Part model, mm, in its own coordinate system. A direction names the side the tool comes from. Round coordinates to 2 decimals unless told otherwise and drop trailing zeros. Loops run counter-clockwise (first coordinate to the right, second up) from the corner with the lowest first, then second, coordinate; pieces in that order, holes last. Notation, with made-up numbers: (9.5, 69) -> (33.5, 69) arc R18 ccw to (33.5, 84) -> close; hole circle Ø7 at (25, -12.75). An arc over 180 degrees is marked (long way). Answer as a JSON object with one key per item and string values. Group by question number.
Autodesk Inventor part; units mm, degrees
ref_plane "YZ Plane" through (0, 0, 0) normal (1, 0, 0) x (0, 1, 0)
ref_plane "XZ Plane" through (0, 0, 0) normal (0, 1, 0) x (-1, 0, 0)
ref_plane "XY Plane" through (0, 0, 0) normal (0, 0, 1) x (1, 0, 0)
sketch "Sketch1" plane through (0, 0, 0) normal (0, 1, 0) x (-1, 0, 0)
  line L0 (0, 0) -> (0, 25.4)
  line L1 (0, 25.4) -> (50.8, 25.4)
  line L2 (50.8, 25.4) -> (50.8, 0)
  line L3 (50.8, 0) -> (0, 0)
  dimension "d0" = 25.4
  dimension "d1" = 50.8
extrude "Plate1" add sketch "Sketch1" along normal blind 3.048
sketch "Sketch2" plane through (-3.048, 0, 0) normal (1, 0, 0) x (0, 1, 0)
  line L0 (0, 25.4) -> (0, 0)
  line L1 (0, 0) -> (76.2, 0)
  line L2 (76.2, 0) -> (76.2, 25.4)
  line L3 (76.2, 25.4) -> (0, 25.4)
edge flange "Flange1" height 76.2 angle 90 thickness 3.048 bend radius 3.048 thickness toward (1, 0, 0) relief tear relief width 3.048 relief depth 1.524 edges at (0, 3.048, 12.7) wall of the first edge with corners at (-3.048, 0, 25.4) (-3.048, 0, 0) (-3.048, 76.2, 0) (-3.048, 76.2, 25.4)
bend "Bend1"
corner "Corner1"
hole "Hole1" at (-3.048, 12.7, 12.7) direction (1, 0, 0) diameter 6.35 end through all
pattern_linear "Rectangular Pattern1" count 3 spacing 25.4 along (0, 1, 0) of "Hole1"
hole "Hole2" at (-12.7, 3.048, 12.7) direction (0, -1, 0) diameter 6.35 end through all
pattern_linear "Rectangular Pattern2" count 2 spacing 25.4 along (-1, 0, 0) of "Hole2"
equation "\"d20\" = Thickness"
equation "\"d32\" = Thickness"
equation "\"d3\" = BendReliefWidth"
equation "\"d4\" = BendReliefDepth"
equation "\"d5\" = MinimumRemnant"
equation "\"d6\" = BendRadius"
equation "\"d9\" = BendRadius"
equation "\"d10\" = CornerReliefSize"
equation "\"d11\" = GapSize"
equation "\"d12\" = JacobiRadiusSize"
equation "\"BendRadius\" = Thickness"
equation "\"BendReliefWidth\" = Thickness"
equation "\"BendReliefDepth\" = 0.5 * Thickness"
equation "\"CornerReliefSize\" = 4 * Thickness"
equation "\"MinimumRemnant\" = 2 * Thickness"
equation "\"TransitionRadius\" = BendRadius"
equation "\"JacobiRadiusSize\" = BendRadius"
equation "\"GapSize\" = Thickness"
equation "\"d2\" = BendRadius"
properties part number "L-Gusset Steel Plate"
Item 1: Band-saw the part on A-A, the plane x = -38.1. List the corners of the cut face in (y, z) (3 decimals), plus the area to 3 significant figures.
Item 2: Band-saw the part on C-C, the plane z = 12.7. List the corners of the cut face in (x, y) (3 decimals), plus the area to 3 significant figures.
Item 3: Band-saw the part on B-B, the plane y = 12.7. List the corners of the cut face in (x, z) (3 decimals), plus the area to 3 significant figures.
Item 4: Two-plate mould, pull along Y, no slides. Class faces 3 (the face through (-1.5, 14.63, 10.18)), 4 (the face through (-2, 76.2, 13)), 5 (the face through (-50.8, 2, 13)), 6 (the face through (-1.503, 61.354, 10.36)): pulls with the +Y half, pulls with the -Y half, needs draft (parallel to the pull), parting line crosses it, or undercut.
Item 5: Band-saw the part on D-D, the plane z = 5.5. List the corners of the cut face in (x, y), plus the area to 3 significant figures.
Item 6: Drill centre lines: line 1 (Y direction, x = -1.75, z = 12.7) (3 decimals); line 2 (Z direction, x = -0.7, y = 38.1) (3 decimals); line 3 (X direction, y = 2, z = 12.7) (3 decimals). Where is each one in solid material? Low to high.
Item 7: Which spindle directions (+Z, -Z, +X, -X, +Y, -Y) get a long thin tool onto all of the face, cutting with end or side? Do faces 1 (the face through (-2.7, 27, 0)), 2 (the face through (-3.048, 41, 15)). Say none if no direction does.
Item 8: Drop flat-ended pins along their axis: pin 1 Ø12.5 at (y, z) = (40.5, 14) entering from -X; pin 2 Ø8 at (x, z) = (-27.5, 16.5) entering from +Y. Give the stop position or say it passes through.
Entries:
{
 "1": {"outline": "(0, 0) -> (3.048, 0) -> (3.048, 9.525) -> (0, 9.525) -> close; (0, 15.875) -> (3.048, 15.875) -> (3.048, 25.4) -> (0, 25.4) -> close", "area": "58.1 mm²"},
 "2": {"outline": "(-50.8, 0) -> (-41.275, 0) -> (-41.275, 3.048) -> (-50.8, 3.048) -> close; (-34.925, 0) -> (-15.875, 0) -> (-15.875, 3.048) -> (-34.925, 3.048) -> close; (-9.525, 0) -> (-6.096, 0) arc R6.096 ccw to (0, 6.096) -> (0, 9.525) -> (-3.048, 9.525) -> (-3.048, 6.096) arc R3.048 cw to (-6.096, 3.048) -> (-9.525, 3.048) -> close; (-3.048, 15.875) -> (0, 15.875) -> (0, 34.925) -> (-3.048, 34.925) -> close; (-3.048, 41.275) -> (0, 41.275) -> (0, 60.325) -> (-3.048, 60.325) -> close; (-3.048, 66.675) -> (0, 66.675) -> (0, 76.2) -> (-3.048, 76.2) -> close", "area": "275 mm²"},
 "3": {"outline": "(-3.048, 0) -> (0, 0) -> (0, 9.525) -> (-3.048, 9.525) -> close; (-3.048, 15.875) -> (0, 15.875) -> (0, 25.4) -> (-3.048, 25.4) -> close", "area": "58.1 mm²"},
 "4": {"face 3": "undercut", "face 4": "pulls with the +Y half", "face 5": "needs draft", "face 6": "undercut"},
 "5": {"outline": "(-50.8, 0) -> (-6.1, 0) arc R6.1 ccw to (0, 6.1) -> (0, 76.2) -> (-3.05, 76.2) -> (-3.05, 6.1) arc R3.05 cw to (-6.1, 3.05) -> (-50.8, 3.05) -> close", "area": "372 mm²"},
 "6": {"line 1": "1.821 to 9.525, 15.875 to 34.925, 41.275 to 60.325, 66.675 to 76.2", "line 2": "0 to 9.525, 15.875 to 25.4", "line 3": "-50.8 to -41.275, -34.925 to -15.875, -9.525 to -1.581"},
 "7": {"face 1": "-Z, +X, -X, +Y, -Y", "face 2": "+Z, -Z, -X, +Y"},
 "8": {"pin 1": "x = -3.05", "pin 2": "y = 3.05"}
}
